Input: part model. Units: mm. Frame: model coordinates. A direction names the side the tool comes from. Round coordinates to 2 decimals unless told otherwise and drop trailing zeros. Write each loop counter-clockwise with the first axis right and the second up, starting at its lowest first coordinate (ties: lowest second). Pieces come first, ordered by that corner, then holes. Notation, with made-up numbers: (36.5, 85.25) -> (71.5, 85.25) arc R14 ccw to (71.5, 95.25) -> close; hole circle Ø11 at (-6.75, -14). An arc over 180 degrees is marked (long way). Write item = value, one per line.
```python
from build123d import *

# Parameters (mm, degrees)
BOSS_EXTRUDE1_DEPTH = 3.5
CUT_EXTRUDE1_DEPTH  = 55.39329676
FILLET10_R          = 2


with BuildPart() as part:
    # Sketch1 → Boss-Extrude1 (new, symmetric)
    with BuildSketch(Plane(origin=(0, 0, 0), x_dir=(0, 0, -1), z_dir=(1, 0, 0))):
        Polygon((0, 0), (0, 15), (6, 31.484864517), (6, 46.484864517), (9, 46.484864517), (9, 30.955883575), (3, 14.471019058), (3, 0), align=None)
    extrude(amount=BOSS_EXTRUDE1_DEPTH, both=True)

    # Sketch2 → Revolve1 (revolve)
    with BuildSketch(Plane(origin=(0, 46.484864517, 0), x_dir=(1, 0, 0), z_dir=(0, 1, 0))):
        with BuildLine():
            Line((0, 2), (0, 9))
            Line((0, 9), (6.062177826, 9))
            ThreePointArc((6.062177826, 9), (7, 5.5), (6.062177826, 2))
            Line((6.062177826, 2), (0, 2))
        make_face()
    revolve(axis=Axis((0, 46.484864517, -2), (0, 0, -1)))

    # Sketch3 → Cut-Revolve1 (revolve, cut)
    with BuildSketch(Plane(origin=(0, 0, 0), x_dir=(0, 0, -1), z_dir=(1, 0, 0))):
        with BuildLine():
            Line((2, 46.484864517), (9, 46.484864517))
            Line((9, 46.484864517), (9, 42.914150302))
            ThreePointArc((9, 42.914150302), (5.5, 41.484864517), (2, 42.914150302))
            Line((2, 42.914150302), (2, 46.484864517))
        make_face()
    revolve(axis=Axis((0, 46.484864517, -2), (0, 0, -1)), mode=Mode.SUBTRACT)

    # Sketch4 → Cut-Extrude1 (cut, through all)
    with BuildSketch(Plane.XY.offset(-2)):
        with BuildLine():
            ThreePointArc((-3.092329219, 48.270221624), (-3.719932076, 50.612467374), (-6.062177826, 49.984864517))
            ThreePointArc((-6.062177826, 49.984864517), (0, 53.484864517), (6.062177826, 49.984864517))
            ThreePointArc((6.062177826, 49.984864517), (3.719932076, 50.612467374), (3.092329219, 48.270221624))
            ThreePointArc((3.092329219, 48.270221624), (0, 50.055578731), (-3.092329219, 48.270221624))
        make_face()
    extrude(amount=-CUT_EXTRUDE1_DEPTH, mode=Mode.SUBTRACT)

    # Fillet10
    fillet10_edges = [part.edges().sort_by_distance(p)[0] for p in [
        (-3.5, 36.245500312, -9),
        (-3.5, 22.713451316, -6),
        (-3.5, 7.235509529, -3),
        (3.5, 22.713451316, -6),
        (0, 30.955883575, -9),
        (0, 14.471019058, -3),
        (0, 0, -3),
        (3.5, 36.245500312, -9),
        (3.5, 7.235509529, -3),
    ]]
    fillet(fillet10_edges, radius=FILLET10_R)


solid = part.part
```
1) Line query: L1, parallel to Z at x = 0, y = 38; L2, parallel to X at y = 26, z = -5. Output: solid intervals per line, ascending. Write a range as from..to.
Solutions:
L1 = -9..-6
L2 = -3.5..3.5
2) First-contact query: P1, Ø2, axis at y = 26, z = -4, coming from the -X side; P2, Ø0.9, axis at x = 0, y = 6.5, coming from the -Z side. Flat tips, straight axial feed; report the tip coordinate or a pass-through.
Solutions:
P1 = -3.5
P2 = -3
3) Cut plane A-A (y = 34). Return the cut outline in (x, z), and give its area (3 significant figures).
Solutions:
outline = (-3.5, -7) arc R2 ccw to (-1.5, -9) -> (1.5, -9) arc R2 ccw to (3.5, -7) -> (3.5, -6) -> (-3.5, -6) -> close
area = 19.3 mm^2
4) Access query for faces 1 (the face through (2.9, 6.96, -2.43)), 2 (the face through (0, 7, 0)), 3 (the face through (0, 42, -2)), 4 (the face through (0, 8, -3)). Directions: +Z, -Z, +X, -X, +Y, -Y. A direction counts if a zero-diameter tool reaches every point of the face in a straight line with its end or side. Return the directions, or none.
Solutions:
face_1 = -Z, +X, -Y
face_2 = +Z, +X, -X, +Y, -Y
face_3 = +Z, +X, -X, +Y
face_4 = -Z, +X, -X, -Y
5) Draft query along Y for faces 5 (the face through (3.5, 20.4, -2.7)), 6 (the face through (0.05, 23.13, -2.96)), 7 (the face through (0.02, 22.82, -6.04)). Return one class per face: +Y half, -Y half, draft (parallel to the pull), parting line (faces both ways), or undercut.
Solutions:
face_5 = draft
face_6 = undercut
face_7 = -Y half
